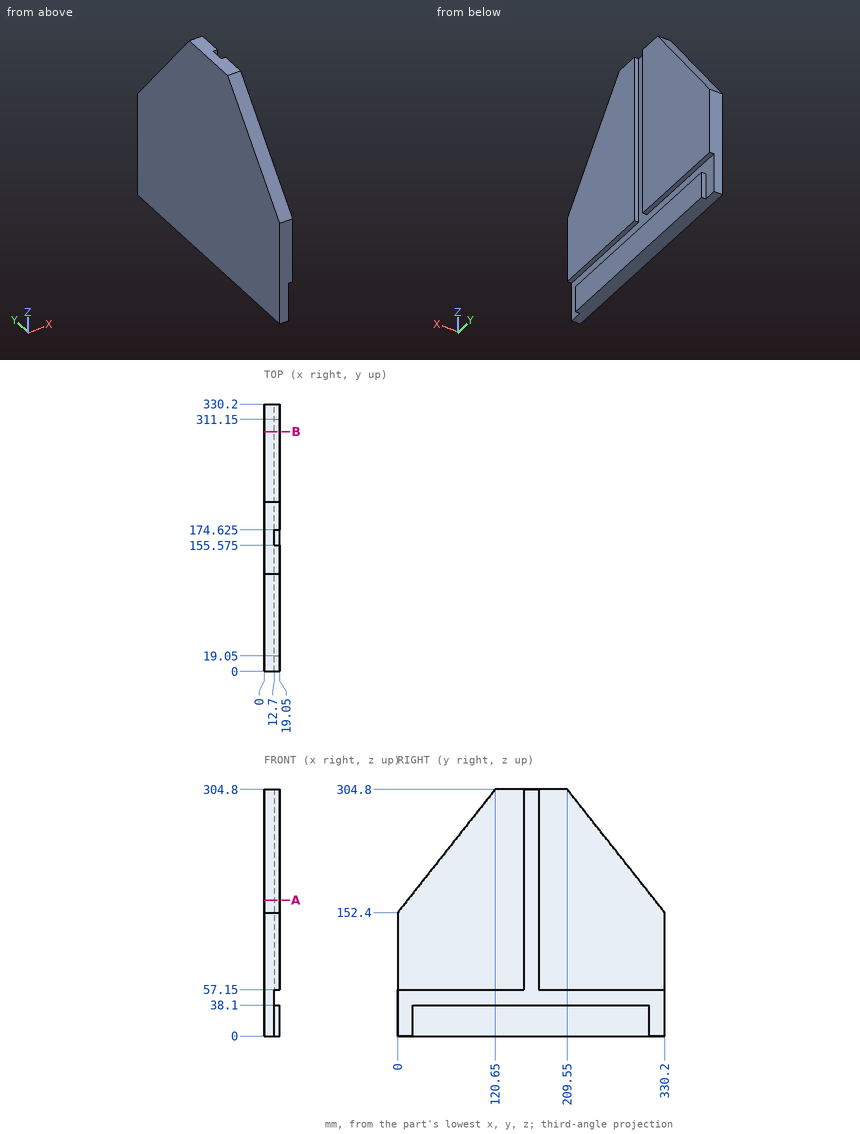
The drawing under review shows one solid part. Ordinate dimensions are in mm from its lowest x, y, z. Coordinates: 2 decimals unless noted, no trailing zeros. Loops run counter-clockwise (first coordinate to the right, second up) from the corner with the lowest first, then second, coordinate; pieces in that order, holes last. Notation, with made-up numbers: M 19.5,89.5 L 60.5,89.5 A26 ccw 60.5,113.5 Z; hole C 26.25,58.25 d1. An arc over 180 degrees is marked long. Use one line per item in the form item = value.
(1) Consider section B-B (y = 296). Write out the cut boundary in (x, z).
Return value:
outline = M 0,0 L 19.05,0 L 19.05,38.1 L 12.7,38.1 L 12.7,57.15 L 19.05,57.15 L 19.05,195.6 L 0,195.6 Z
(2) Consider section A-A (z = 168). Write out the cut boundary in (x, y) (3 decimals), and give its area (3 significant figures).
Return value:
outline = M 0,12.35 L 19.05,12.35 L 19.05,155.575 L 12.7,155.575 L 12.7,174.625 L 19.05,174.625 L 19.05,317.85 L 0,317.85 Z
area = 5,700 mm2
(3) Clearance check with flat-ended pins moving along their axes: P1, Ø7, axis at x = 16, z = 242, coming from the -Y side; P2, Ø8, axis at x = 2.5, z = 254, coming from the +Y side; P3, Ø1.9, axis at x = 17.5, z = 10, coming from the +Y side. State where each tip first meets the part, or that it passes through.
Return value:
P1 = 68.16
P2 = 252.93
P3 = 311.15
(4) For line 1 along Z through (x, y) = (18, 187); line 2 along Y through (x, z) = (14.5, 69.5) (3 decimals); line 3 along Z through (x, y) = (13.25, 30), list the stretches that pass through material, from the lowest coordinate up. Write a range as from..to.
Return value:
line_1 = 0..38.1, 57.15..304.8
line_2 = 0..155.575, 174.625..330.2
line_3 = 0..38.1, 57.15..190.29
